from build123d import *

# Parameters (mm, degrees)
SKETCH019_W             = 74
SKETCH019_H             = 16
PAD013_DEPTH            = 1
SKETCH003_W             = 1
SKETCH003_H             = 16
PAD002_DEPTH            = 10
PAD002_FACE6_W          = 16
PAD002_FACE6_H          = 72
PAD012_DEPTH            = 9
SKETCH021_W             = 66
SKETCH021_H             = 16
POCKET008_DEPTH         = 9
SKETCH023_R             = 2.5
PAD010_DEPTH            = 1.9
SKETCH024_R             = 1.05
POCKET007_DEPTH         = 5
BODY005_PLACEMENT_ANGLE = 90


with BuildPart() as part:
    # Sketch019 → Pad013 (new body)
    with BuildSketch(Plane.XY):
        with Locations((35, 7)):
            Rectangle(SKETCH019_W, SKETCH019_H)
    extrude(amount=PAD013_DEPTH)

    # Sketch003 (on Face6 of Pad013) → Pad002 (join)
    with BuildSketch(Plane.XY.offset(1)):
        with Locations((-1.5, 7)):
            Rectangle(SKETCH003_W, SKETCH003_H)
        with Locations((71.5, 7)):
            Rectangle(SKETCH003_W, SKETCH003_H)
    extrude(amount=PAD002_DEPTH)

    # Pad002 Face6 → Pad012 (add)
    with BuildSketch(Plane(origin=(35, 7, 1), x_dir=(0, 1, 0), z_dir=(0, 0, 1))):
        Rectangle(PAD002_FACE6_W, PAD002_FACE6_H)
    extrude(amount=PAD012_DEPTH)

    # Sketch021 (on Face13 of Pad012) → Pocket008 (cut)
    with BuildSketch(Plane.XY.offset(10)):
        with Locations((35, 7)):
            Rectangle(SKETCH021_W, SKETCH021_H)
    extrude(amount=-POCKET008_DEPTH, mode=Mode.SUBTRACT)

    # Sketch023 (on Face7 of Pocket008) → Pad010 (join)
    with BuildSketch(Plane.XY.offset(1)):
        with Locations((34, 9)):
            Circle(SKETCH023_R)
    extrude(amount=PAD010_DEPTH)

    # Sketch024 (on Face26 of Pad010) → Pocket007 (cut)
    with BuildSketch(Plane.XY.offset(2.9)):
        with Locations((34, 9)):
            Circle(SKETCH024_R)
    extrude(amount=-POCKET007_DEPTH, mode=Mode.SUBTRACT)


with BuildPart() as part_1:
    # Body005 placement: moved
    add(part.part.moved(Location((97, 2, -10))).rotate(Axis((97, 2, -10), (0, 0, 1)), BODY005_PLACEMENT_ANGLE))


solid = part_1.part
Here's how the part is built. I have some questions about the finished solid (model axes, mm). A direction names the side the tool comes from. Coordinates: 2 decimals unless noted, no trailing zeros. Order: outer loops, then holes, each group sorted by start corner. A loop starts at its lowest first (then second) coordinate and runs counter-clockwise, first axis right, second up. Notation, with made-up numbers: (86.5, 72.25) -> (121.5, 72.25) arc R10 cw to (121.5, 84.25) -> close; hole circle Ø6 at (89, 55). An arc over 180 degrees is marked (long way). Answer in a Markdown table with one row per item.
(1) I want a section at D-D on y = 36. List the corners of the cut face in (x, z) for me, then the cut area to 3 significant figures.
Answer key:
| item | result |
|---|---|
| outline | (82, -10) -> (86.95, -10) -> (86.95, -7.1) -> (85.5, -7.1) -> (85.5, -9) -> (82, -9) -> close; (89.05, -10) -> (98, -10) -> (98, -9) -> (90.5, -9) -> (90.5, -7.1) -> (89.05, -7.1) -> close |
| area | 19.4 mm^2 |
(2) Please list where these lines run through material, in increasing order: probe 1 along Y at (x, z) = (88, -8.6); probe 2 along Y at (x, z) = (90.5, -5.25); probe 3 along Y at (x, z) = (88, -9.3).
Answer key:
| item | result |
|---|---|
| probe 1 | 0 to 4, 33.5 to 34.95, 37.05 to 38.5, 70 to 74 |
| probe 2 | 0 to 4, 70 to 74 |
| probe 3 | 0 to 34.95, 37.05 to 74 |
(3) Thinking about a two-plate mould opening in X: for faces 4 (the face through (86.96, 35.86, -8.53)), 5 (the face through (98, 42.7, -9.4)), 6 (the face through (90, 4, -4)), which applies, +X half, -X half, draft (parallel to the pull), parting line (faces both ways), or undercut?
Answer key:
| item | result |
|---|---|
| face 4 | undercut |
| face 5 | +X half |
| face 6 | draft |
(4) I want a section at C-C on z = -8.25. List the corners of the cut face in (x, y) for me, then the cut area to 3 significant figures.
Answer key:
| item | result |
|---|---|
| outline | (82, 0) -> (98, 0) -> (98, 4) -> (82, 4) -> close; (82, 70) -> (98, 70) -> (98, 74) -> (82, 74) -> close; circle Ø5 at (88, 36); hole circle Ø2.1 at (88, 36) |
| area | 144 mm^2 |
(5) On a 3-axis mill with a long thin cutter (end or side, diameter ignored), from which of +Z, -Z, +X, -X, +Y, -Y can I reach the whole of each face in a straight line? I mean faces 1 (the face through (90, 2, 0)), 2 (the face through (87.249, 38.385, -8.063)), 3 (the face through (90, 74, -5)). Say none if no direction works.
Answer key:
| item | result |
|---|---|
| face 1 | +Z, +X, -X |
| face 2 | +Z |
| face 3 | +Z, -Z, +X, -X, +Y |
(6) Will these pins go through, and if not, where does the flat tip stop? pin 1 Ø1.5 at (x, y) = (87.5, 36.5) entering from +Z; pin 2 Ø0.9 at (x, y) = (90.5, 3) entering from +Z; pin 3 Ø4 at (y, z) = (40, -5) entering from -X; pin 4 Ø2.5 at (x, y) = (88, 36) entering from -Z.
Answer key:
| item | result |
|---|---|
| pin 1 | z = -7.1 |
| pin 2 | z = 0 |
| pin 3 | through |
| pin 4 | z = -10 |
(7) I want a section at A-A on z = -2.5. List the corners of the cut face in (x, y) for me.
Answer key:
| item | result |
|---|---|
| outline | (82, 0) -> (98, 0) -> (98, 4) -> (82, 4) -> close; (82, 70) -> (98, 70) -> (98, 74) -> (82, 74) -> close |
(8) I want a section at B-B on x = 88. List the corners of the cut face in (y, z) for me.
Answer key:
| item | result |
|---|---|
| outline | (0, -10) -> (34.95, -10) -> (34.95, -7.1) -> (33.5, -7.1) -> (33.5, -9) -> (4, -9) -> (4, 0) -> (1, 0) -> (1, 1) -> (0, 1) -> close; (37.05, -10) -> (74, -10) -> (74, 1) -> (73, 1) -> (73, 0) -> (70, 0) -> (70, -9) -> (38.5, -9) -> (38.5, -7.1) -> (37.05, -7.1) -> close |
